Geometry check sheet. Reference: the model listing, model coordinates, mm. Coordinates: 2 decimals unless noted, no trailing zeros. Write each loop counter-clockwise with the first axis right and the second up, starting at its lowest first coordinate (ties: lowest second). Pieces come first, ordered by that corner, then holes. Notation, with made-up numbers: M 65.25,81 L 116.25,81 A21 cw 116.25,118 Z; hole C 84.5,60 d9. An arc over 180 degrees is marked long. Answer as a JSON object with one key per item and string values. Group by question number.
```python
from build123d import *

# Parameters (mm, degrees)
SKETCH1_R           = 1.324438001
SKETCH1_R_2         = 1.324206598
SKETCH1_R_3         = 1.497599193
BOSS_EXTRUDE1_DEPTH = 3.175


with BuildPart() as part:
    # Sketch1 → Boss-Extrude1 (new body)
    with BuildSketch(Plane(origin=(0, 0, 0), x_dir=(1, 0, 0), z_dir=(0, 1, 0))):
        with BuildLine():
            ThreePointArc((-9.665902261, -17.771312034), (-6.897981116, -23.219424369), (-2.001997786, -19.562559221))
            add(Edge.make_bspline(
                [(17.513490591, 19.383376385), (6.94674585, 8.875130126), (0.096552729, -4.795463741), (-2.001997786, -19.562559221)],
                knots=[13, 13, 13, 13, 14, 14, 14, 14], degree=3))
            ThreePointArc((17.513490591, 19.383376385), (17.70603035, 24.895348878), (12.202596033, 25.257458036))
            ThreePointArc((12.202596033, 25.257458036), (5.943668971, 22.793339165), (-0.51448442, 24.674377327))
            ThreePointArc((-0.51448442, 24.674377327), (-8.990035225, 25.434433607), (-9.750091506, 16.958882802))
            add(Edge.make_bspline(
                [(-9.665902261, -17.771312034), (-3.58318049, 6.010156861), (-6.384705359, 12.673352049), (-9.750091506, 16.958882802)],
                knots=[4, 4, 4, 4, 5, 5, 5, 5], degree=3))
        make_face()
        with Locations(Location((-5.989030334, -19.330451358, 0), (0, 0, 270))):
            Circle(SKETCH1_R, mode=Mode.SUBTRACT)
        with Locations(Location((14.767597212, 22.238642776, 0), (0, 0, 270))):
            Circle(SKETCH1_R_2, mode=Mode.SUBTRACT)
        with Locations(Location((-5.132287963, 20.816630064, 0), (0, 0, 270))):
            Circle(SKETCH1_R_3, mode=Mode.SUBTRACT)
    extrude(amount=BOSS_EXTRUDE1_DEPTH)


solid = part.part
```
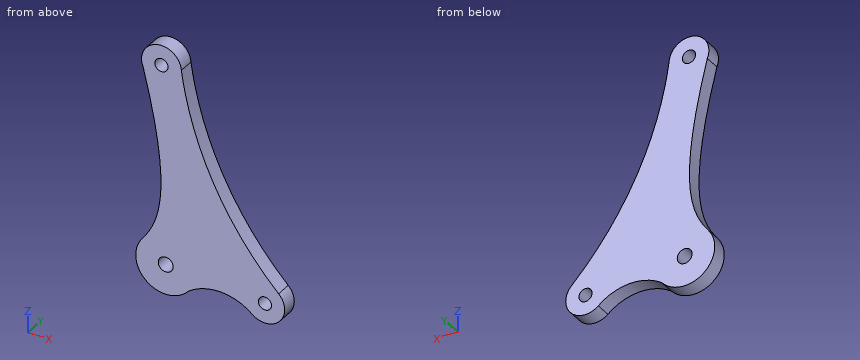
1) Section check A-A (z = -21.5). Record the cut outline in (x, y) (1 decimal), then the cut area to 3 significant figures.
2) Go/stop test with flat-tipped pins: pin 1 Ø1.5 at (y, z) = (0.5, -13.5) entering from -X; pin 2 Ø5 at (x, z) = (1, -6.5) entering from -Y. Record where each tip stops, or that it passes through.
3) Section check B-B (y = 0.9). State how many separate pieces and enclosed holes the cut face has, then the cut area to 3 significant figures.
4) Material ranges on probe 1 along X at (y, z) = (1.5, 6); probe 2 along X at (y, z) = (2, -9); probe 3 along Z at (x, y) = (10.5, 1.55), recorded low to high. Write a range as [from, to].
Entries:
{
 "1": {"outline": "M -11.1,0 L -6.5,0 L -6.5,3.2 L -11.1,3.2 Z; M -3.8,0 L 13.7,0 L 13.7,3.2 L -3.8,3.2 Z; M 15.9,0 L 18.7,0 L 18.7,3.2 L 15.9,3.2 Z", "area": "79.1 mm^2"},
 "2": {"pin 1": "x = -8", "pin 2": "y = 0"},
 "3": {"separate pieces": "1", "enclosed holes": "3", "area": "660 mm^2"},
 "4": {"probe 1": "[-7.11, 1.36]", "probe 2": "[-6.39, 8.95]", "probe 3": "[-24.08, -11.21]"}
}
